For this review, take the finished solid that the model builds, in its own axes (mm). Face numbers are marked on the shaded views. A direction names the side the tool comes from. Give positions to 0.01 mm unless a question says otherwise; leave off trailing zeros. Order: outer loops, then holes, each group sorted by start corner. A loop starts at its lowest first (then second) coordinate and runs counter-clockwise, first axis right, second up. Notation, with made-up numbers: (-28, -29) - (12, -29) arc R20 ccw to (12, -15) - close; hole circle Ø4 at (16.25, 66.5). An arc over 180 degrees is marked (long way). Use a Markdown table: item, result. Add a question column.
1) We need section C-C on y = -3.75. Write out the cut boundary in (x, z).
2) We need section D-D on x = 0. Give the number of separate pieces and of enclosed holes in the cut face, then the cut area to 3 significant figures.
3) Wall thickness on L1, parallel to Y at x = 13, z = 3.1; L2, parallel to Y at x = 11, z = 0.25; L3, parallel to Z at x = 3.5, y = 1: over which ranges is each line inside the solid? List them lowest first.
4) Machinability: for the marked faces 1 and 2, which of the approach directions +Z, -Z, +X, -X, +Y, -Y give a long, thin tool a straight path to every point of the face, cutting with its end or side? Answer none if there is none.
5) Clearance check with flat-ended pins moving along their axes: P1, Ø0.7, axis at x = 9.09, y = -5.25, coming from the +Z side; P2, Ø10, axis at x = 11.5, y = 2, coming from the -Z side; P3, Ø2, axis at x = 5, y = -6, coming from the -Z side; P4, Ø2, axis at x = -12.5, z = 3, coming from the +Y side. State where each tip first meets the part, or that it passes through.
6) Mouldability with a two-part tool opening along Y and no side actions: class the marked faces 3, 4 and 5 as released by +Y, released by -Y, zero draft, split by the parting line, or undercut.
7) We need section A-A on y = 0. Write out the cut boundary in (x, z) (3 decimals), then the cut area to 3 significant figures.
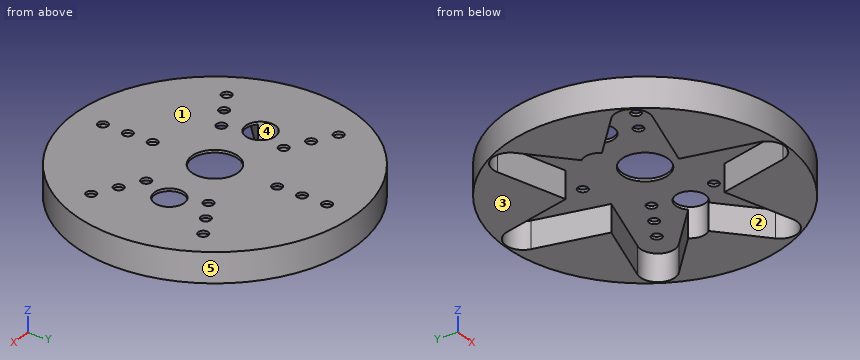
```python
from build123d import *

# Parameters (mm, degrees)
SKETCH1_R               = 17
BOSS_EXTRUDE1_DEPTH     = 3.6
CAVITY1_OUTLINE_R       = 3.15
CAVITY1_DEPTH           = 3.283595969
CAVITY1_START           = 1.183595969
CAVITY1_2_OUTLINE_R     = 3.15
CAVITY1_2_OUTLINE_R_2   = 1.575
CAVITY1_2_DEPTH         = 2.1
SKETCH2_R               = 0.6
CUT_EXTRUDE1_DEPTH      = 10
CIRPATTERN1_COUNT       = 6
SKETCH3_R               = 4.596048158
CUT_EXTRUDE2_DEPTH      = 3.283595969
CUT_EXTRUDE3_DEPTH      = 25.309668858
CUT_EXTRUDE3_DEPTH_BACK = 25.309668858
SKETCH4_R               = 2.8
SKETCH6_R               = 1.8
CUT_EXTRUDE4_DEPTH      = 10


# Read off the part's stored shape, not the designer's step: Cavity1
with BuildPart() as part:
    # Sketch1 → Boss-Extrude1 (new body)
    with BuildSketch(Plane.XY):
        Circle(SKETCH1_R)
    extrude(amount=BOSS_EXTRUDE1_DEPTH)

    # Cavity1 outline → Cavity1 (cut)
    with BuildSketch(Plane.XY):
        with BuildLine():
            Line((3.9375, 6.819950055), (2.048148228, 15.163776711))
            ThreePointArc((2.048148228, 15.163776711), (0, 16.8), (-2.048148228, 15.163776711))
            Line((-2.048148228, 15.163776711), (-3.9375, 6.819950055))
            Line((-3.9375, 6.819950055), (-12.108141735, 9.355636751))
            ThreePointArc((-12.108141735, 9.355636751), (-14.549226784, 8.4), (-14.156289963, 5.80813996))
            Line((-14.156289963, 5.80813996), (-7.875, 0))
            Line((-7.875, 0), (-14.156289963, -5.80813996))
            ThreePointArc((-14.156289963, -5.80813996), (-14.549226784, -8.4), (-12.108141735, -9.355636751))
            Line((-12.108141735, -9.355636751), (-3.9375, -6.819950055))
            Line((-3.9375, -6.819950055), (-2.048148228, -15.163776711))
            ThreePointArc((-2.048148228, -15.163776711), (0, -16.8), (2.048148228, -15.163776711))
            Line((2.048148228, -15.163776711), (3.9375, -6.819950055))
            Line((3.9375, -6.819950055), (12.108141735, -9.355636751))
            ThreePointArc((12.108141735, -9.355636751), (14.549226784, -8.4), (14.156289963, -5.80813996))
            Line((14.156289963, -5.80813996), (7.875, 0))
            Line((7.875, 0), (14.156289963, 5.80813996))
            ThreePointArc((14.156289963, 5.80813996), (14.549226784, 8.4), (12.108141735, 9.355636751))
            Line((12.108141735, 9.355636751), (3.9375, 6.819950055))
        make_face()
        Circle(CAVITY1_OUTLINE_R, mode=Mode.SUBTRACT)
    extrude(amount=CAVITY1_DEPTH, mode=Mode.SUBTRACT)

    # Cavity1 2 outline → Cavity1 2 (cut)
    with BuildSketch(Plane.XY.offset(CAVITY1_START)):
        Circle(CAVITY1_2_OUTLINE_R)
        Circle(CAVITY1_2_OUTLINE_R_2, mode=Mode.SUBTRACT)
    extrude(amount=CAVITY1_2_DEPTH, mode=Mode.SUBTRACT)

    # Sketch2 → Cut-Extrude1 (cut)
    with BuildSketch(Plane(origin=(0, 0, 0), x_dir=(-1, 0, 0), z_dir=(0, 0, -1))):
        with Locations(Location((0, 13.5, 0), (0, 0, 180))):
            Circle(SKETCH2_R)
        with Locations(Location((0, 10.5, 0), (0, 0, 180))):
            Circle(SKETCH2_R)
        with Locations(Location((0, 7.5, 0), (0, 0, 180))):
            Circle(SKETCH2_R)
    cut_extrude1 = extrude(amount=-CUT_EXTRUDE1_DEPTH, mode=Mode.SUBTRACT)

    # CirPattern1: Cut-Extrude1 ×6 about axis
    cirpattern1_axis = Axis((0, 0, 0), (0, 0, 1))
    for i in range(1, CIRPATTERN1_COUNT):
        add(cut_extrude1.rotate(cirpattern1_axis, i * 360 / CIRPATTERN1_COUNT), mode=Mode.SUBTRACT)

    # Sketch3 → Cut-Extrude2 (cut)
    with BuildSketch(Plane(origin=(0, 0, 0), x_dir=(-1, 0, 0), z_dir=(0, 0, -1))):
        Circle(SKETCH3_R)
    extrude(amount=-CUT_EXTRUDE2_DEPTH, mode=Mode.SUBTRACT)

    # Sketch4 → Cut-Extrude3 (cut, two sides: drawn at the far end of the back side and taken through both)
    with BuildSketch(Plane.XY.offset(3.6).offset(-CUT_EXTRUDE3_DEPTH_BACK)):
        Circle(SKETCH4_R)
    extrude(amount=CUT_EXTRUDE3_DEPTH + CUT_EXTRUDE3_DEPTH_BACK, mode=Mode.SUBTRACT)

    # Sketch6 → Cut-Extrude4 (cut)
    with BuildSketch(Plane(origin=(0, 0, 0), x_dir=(-1, 0, 0), z_dir=(0, 0, -1))):
        with Locations(Location((-7.875, 0, 0), (0, 0, 137.241269402))):
            Circle(SKETCH6_R)
        with Locations(Location((7.875, 0, 0), (0, 0, 42.758730598))):
            Circle(SKETCH6_R)
    extrude(amount=-CUT_EXTRUDE4_DEPTH, mode=Mode.SUBTRACT)


solid = part.part
```
Checked values:
| question | item | result |
|---|---|---|
| 1 | outline | (-16.58, 0) - (-11.93, 0) - (-11.93, 3.28) - (-7.1, 3.28) - (-7.1, 3.6) - (-16.58, 3.6) - close; (-5.9, 3.28) - (5.9, 3.28) - (5.9, 3.6) - (-5.9, 3.6) - close; (7.1, 3.28) - (11.93, 3.28) - (11.93, 0) - (16.58, 0) - (16.58, 3.6) - (7.1, 3.6) - close |
| 2 | separate pieces | 8 |
| 2 | enclosed holes | 0 |
| 2 | area | 8.02 mm² |
| 3 | L1 | -10.95 to -9.43, -4.74 to 4.74, 9.43 to 10.95 |
| 3 | L2 | -12.96 to -9.01, -2.89 to 2.89, 9.01 to 12.96 |
| 3 | L3 | 3.28 to 3.6 |
| 4 | face 1 | +Z, +X, -X, +Y, -Y |
| 4 | face 2 | -Z |
| 5 | P1 | through |
| 5 | P2 | z = 0 |
| 5 | P3 | z = 3.28 |
| 5 | P4 | y = 12.52 |
| 6 | face 3 | zero draft |
| 6 | face 4 | undercut |
| 6 | face 5 | split by the parting line |
| 7 | outline | (-17, 0) - (-9.675, 0) - (-9.675, 3.6) - (-17, 3.6) - close; (-6.075, 3.284) - (-2.8, 3.284) - (-2.8, 3.6) - (-6.075, 3.6) - close; (2.8, 3.284) - (6.075, 3.284) - (6.075, 3.6) - (2.8, 3.6) - close; (9.675, 0) - (17, 0) - (17, 3.6) - (9.675, 3.6) - close |
| 7 | area | 54.8 mm² |
